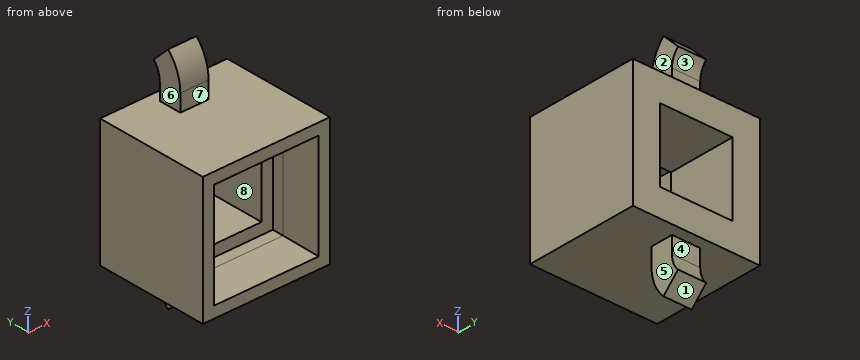
```python
from build123d import *

# Parameters (mm, degrees)
SKETCH1_W           = 22.5
SKETCH1_H           = 22.5
BOSS_EXTRUDE1_DEPTH = 20
SKETCH5_W           = 5
SKETCH5_H           = 4
SKETCH3_W           = 18.5
SKETCH3_H           = 18.5
CUT_EXTRUDE5_DEPTH  = 6
CUT_EXTRUDE5_TAPER  = 8
SKETCH14_W          = 16.813509984
SKETCH14_H          = 16.813509984
CUT_EXTRUDE6_DEPTH  = 2
CUT_EXTRUDE7_REACH  = 14
SKETCH15_W          = 12.813509984
SKETCH15_H          = 12.813509984


with BuildPart() as part:
    # Sketch1 → Boss-Extrude1 (new body)
    with BuildSketch(Plane(origin=(0, 0, 0), x_dir=(1, 0, 0), z_dir=(0, 1, 0))):
        Rectangle(SKETCH1_W, SKETCH1_H)
    extrude(amount=BOSS_EXTRUDE1_DEPTH)

    # Sweep1: sweep along a path in Sketch6
    with BuildLine(Plane(origin=(0, 0, 0), x_dir=(0, 0, -1), z_dir=(1, 0, 0))) as sweep1_path:
        Line((11.25, 16), (14.25, 16))
        ThreePointArc((14.25, 16), (16.546100594, 16.456722805), (18.492640687, 17.757359313))
    # Sketch5 → Sweep1 (sweep)
    with BuildSketch(Plane(origin=(0, 0, -11.25), x_dir=(-1, 0, 0), z_dir=(0, 0, -1))):
        with Locations((0, 16)):
            Rectangle(SKETCH5_W, SKETCH5_H)
    sweep1 = sweep(path=sweep1_path.line)

    # Mirror1: Sweep1 across plane
    add(sweep1.mirror(Plane.XY))

    # Sketch3 → Cut-Extrude5 (cut)
    with BuildSketch(Plane.XZ):
        Rectangle(SKETCH3_W, SKETCH3_H)
    extrude(amount=-CUT_EXTRUDE5_DEPTH, taper=CUT_EXTRUDE5_TAPER, mode=Mode.SUBTRACT)

    # Sketch14 → Cut-Extrude6 (cut)
    with BuildSketch(Plane.XZ.offset(-6)):
        Rectangle(SKETCH14_W, SKETCH14_H)
    extrude(amount=-CUT_EXTRUDE6_DEPTH, mode=Mode.SUBTRACT)

    # Sketch15 → Cut-Extrude7 (cut, up to next)
    with BuildSketch(Plane.XZ.offset(-8), mode=Mode.PRIVATE) as cut_extrude7_sk1:
        Rectangle(SKETCH15_W, SKETCH15_H)
    cut_extrude7_tool1 = extrude(cut_extrude7_sk1.sketch, amount=-CUT_EXTRUDE7_REACH, mode=Mode.PRIVATE) & part.part
    add(cut_extrude7_tool1.solids().sort_by_distance((0, 8, 0))[0], mode=Mode.SUBTRACT)


solid = part.part
```
Part model, mm, in its own coordinate system. Face numbers are marked on the shaded views. A direction names the side the tool comes from. Coordinates: 2 decimals unless noted, no trailing zeros. Write each loop counter-clockwise with the first axis right and the second up, starting at its lowest first coordinate (ties: lowest second). Pieces come first, ordered by that corner, then holes.
Item 1: Which spindle directions (+Z, -Z, +X, -X, +Y, -Y) get a long thin tool onto all of the face, cutting with end or side? Do the marked faces 4, 5, 6, 7 and 8. Say none if no direction does.
Item 2: Slice it at B-B (y = 16.75). Write the cut outline in (x, z).
Item 3: Slice it at C-C (z = 12.5). Write the cut outline in (x, y), and give its area (3 significant figures).
Item 4: Mould opens along Z. For the marked faces 1, 2 and 3 say: released by +Z, released by -Z, zero draft, split by the parting line, or undercut.
Item 5: Pin check, flat tips, straight feed: pin 1 (1.6 mm diameter, centred on y = 16, z = 15.5, fed in from +X); pin 2 (3 mm diameter, centred on x = -8.5, z = -6.5, fed in from -Y); pin 3 (0.9 mm diameter, centred on x = -1, z = 12, fed in from +Y); pin 4 (10 mm diameter, centred on x = 5.5, y = 6, fed in from -Z). Stop position of each tip, or through.
Item 6: Slice it at A-A (y = 8.5). Write the cut outline in (x, z).
Item 7: Probe line 1 (Z direction, x = 0.25, y = 9); line 2 (Z direction, x = -7.5, y = 15.5); line 3 (Y direction, x = -7, z = -7). List the from-to ranges inside material, lowest first.
Results found:
1. face 4: +X, -X, +Y
1. face 5: -Z, +X, +Y, -Y
1. face 6: +Z, -X, +Y, -Y
1. face 7: +Z, +X, -X, -Y
1. face 8: +Y, -Y
2. outline: (-11.25, -11.25) - (-2.5, -11.25) - (-2.5, -19.5) - (2.5, -19.5) - (2.5, -11.25) - (11.25, -11.25) - (11.25, 11.25) - (2.5, 11.25) - (2.5, 19.5) - (-2.5, 19.5) - (-2.5, 11.25) - (-11.25, 11.25) - close; hole (-6.41, -6.41) - (6.41, -6.41) - (6.41, 6.41) - (-6.41, 6.41) - close
3. outline: (-2.5, 14) - (2.5, 14) - (2.5, 18) - (-2.5, 18) - close
3. area: 20.0 mm2
4. face 1: released by -Z
4. face 2: zero draft
4. face 3: undercut
5. pin 1: stops at x = 2.5
5. pin 2: stops at y = 0
5. pin 3: stops at y = 18
5. pin 4: stops at z = -11.25
6. outline: (-11.25, -11.25) - (11.25, -11.25) - (11.25, 11.25) - (-11.25, 11.25) - close; hole (-6.41, -6.41) - (6.41, -6.41) - (6.41, 6.41) - (-6.41, 6.41) - close
7. line 1: z = -11.25 to -6.41, 6.41 to 11.25
7. line 2: z = -11.25 to 11.25
7. line 3: y = 8 to 20
